from build123d import *

# Parameters (mm, degrees)
SKETCH_1_W          = 30
SKETCH_1_H          = 25
EXTRUDE_1_DEPTH     = 10
SKETCH_2_R          = 4
CUT_EXTRUDE_1_DEPTH = 41.311288741
SKETCH_3_R          = 1.5
CUT_EXTRUDE_2_DEPTH = 41.311288741


with BuildPart() as part:
    # 스케치1 → 보스-돌출1 (new body)
    with BuildSketch(Plane(origin=(0, 0, 0), x_dir=(0, 0, -1), z_dir=(1, 0, 0))):
        with Locations((15, 12.5)):
            Rectangle(SKETCH_1_W, SKETCH_1_H)
    extrude(amount=EXTRUDE_1_DEPTH)

    # 스케치2 → 컷-돌출1 (cut, through all)
    with BuildSketch(Plane(origin=(0, 25, 0), x_dir=(1, 0, 0), z_dir=(0, 1, 0))):
        with Locations((10, 15)):
            Circle(SKETCH_2_R)
    extrude(amount=-CUT_EXTRUDE_1_DEPTH, mode=Mode.SUBTRACT)

    # 스케치3 → 컷-돌출2 (cut, through all)
    with BuildSketch(Plane(origin=(10, 0, 0), x_dir=(0, 0, -1), z_dir=(1, 0, 0))):
        with Locations((5.5, 18.75)):
            Circle(SKETCH_3_R)
        with Locations(Location((24.5, 18.75, 0), (0, 0, 180))):
            Circle(SKETCH_3_R)
        with Locations(Location((5.5, 6.25, 0), (0, 0, 180))):
            Circle(SKETCH_3_R)
        with Locations((24.5, 6.25)):
            Circle(SKETCH_3_R)
    extrude(amount=-CUT_EXTRUDE_2_DEPTH, mode=Mode.SUBTRACT)


solid = part.part
Design review of the part built by this model. Coordinates are the model's own, in mm. Coordinates: 2 decimals unless noted, no trailing zeros. Write each loop counter-clockwise with the first axis right and the second up, starting at its lowest first coordinate (ties: lowest second). Pieces come first, ordered by that corner, then holes. Notation, with made-up numbers: (-17, -17) - (23, -17) arc R24 ccw to (23, 10) - close; hole circle Ø3 at (-27.75, -1.75). An arc over 180 degrees is marked (long way). One line per item, written item: value.
1) Add section D-D (x = 9). State the section outline as (y, z) points.
Answer sheet:
outline: (0, -30) - (25, -30) - (25, -18.87) - (0, -18.87) - close; (0, -11.13) - (25, -11.13) - (25, 0) - (0, 0) - close; hole circle Ø3 at (6.25, -24.5); hole circle Ø3 at (6.25, -5.5); hole circle Ø3 at (18.75, -24.5); hole circle Ø3 at (18.75, -5.5)
2) Add section B-B (y = 6.25). State the section outline as (x, z) points.
Answer sheet:
outline: (0, -30) - (10, -30) - (10, -26) - (0, -26) - close; (0, -23) - (10, -23) - (10, -19) arc R4 cw to (10, -11) - (10, -7) - (0, -7) - close; (0, -4) - (10, -4) - (10, 0) - (0, 0) - close
3) Insertion check: pin 1 (5 mm diameter, centred on x = 9, y = 22, fed in from +Z); pin 2 (2.5 mm diameter, centred on y = 18.75, z = -24.5, fed in from -X); pin 3 (1 mm diameter, centred on y = 15, z = -12.5, fed in from +X). Each pin has a flat end and moves straight along its axis. Give the tip position at first contact, or say it passes through.
Answer sheet:
pin 1: stops at z = 0
pin 2: passes through
pin 3: stops at x = 7.35
4) Mouldability with a two-part tool opening along Z and no side actions: class faces 1 (the face through (5, 12, -30)), 2 (the face through (10, 13, -24)), 3 (the face through (5.1, 6.3, -23)) as +Z half, -Z half, draft (parallel to the pull), parting line (faces both ways), or undercut.
Answer sheet:
face 1: -Z half
face 2: draft
face 3: undercut
5) To check wall thickness, follow probe 1 along Y at (x, z) = (8, -5.5); probe 2 along Z at (x, y) = (5.5, 19.75); probe 3 along X at (y, z) = (3.75, -14.75). State the ranges of each line that lie inside material, in increasing order.
Answer sheet:
probe 1: y = 0 to 4.75, 7.75 to 17.25, 20.25 to 25
probe 2: z = -30 to -25.62, -23.38 to -6.62, -4.38 to 0
probe 3: x = 0 to 6.01
6) Add section C-C (z = -5). State the section outline as (x, y) points, plus the area to 3 significant figures.
Answer sheet:
outline: (0, 0) - (10, 0) - (10, 4.84) - (0, 4.84) - close; (0, 7.66) - (10, 7.66) - (10, 17.34) - (0, 17.34) - close; (0, 20.16) - (10, 20.16) - (10, 25) - (0, 25) - close
area: 193 mm2
7) Add section A-A (x = 4). State the section outline as (y, z) points.
Answer sheet:
outline: (0, -30) - (25, -30) - (25, 0) - (0, 0) - close; hole circle Ø3 at (6.25, -24.5); hole circle Ø3 at (6.25, -5.5); hole circle Ø3 at (18.75, -24.5); hole circle Ø3 at (18.75, -5.5)
